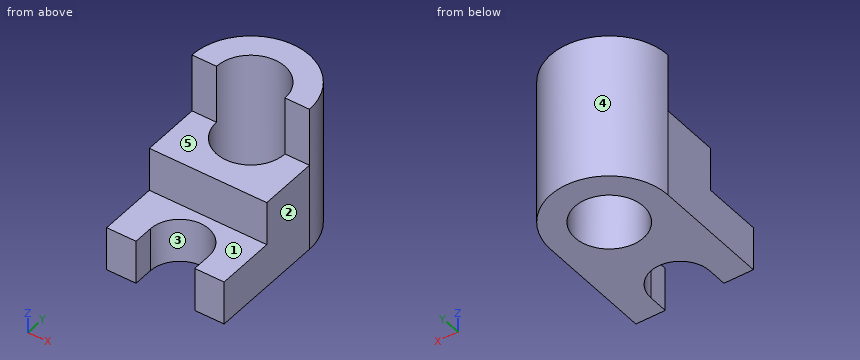
```python
from build123d import *

# Parameters (mm, degrees)
SKETCH1_R           = 3.5
BOSS_EXTRUDE1_DEPTH = 15
CUT_EXTRUDE1_DEPTH  = 15


with BuildPart() as part:
    # Sketch1 → Boss-Extrude1 (new body)
    with BuildSketch(Plane.XY):
        with BuildLine():
            Line((-6, 6), (-6, -6))
            Line((-6, -6), (-3, -6))
            Line((-3, -6), (-3, -3.996197441))
            ThreePointArc((-3, -3.996197441), (0, -0.996197441), (3, -3.996197441))
            Line((3, -3.996197441), (3, -6))
            Line((3, -6), (6, -6))
            Line((6, -6), (6, 6))
            ThreePointArc((6, 6), (0, 12), (-6, 6))
        make_face()
        with Locations((0, 6)):
            Circle(SKETCH1_R, mode=Mode.SUBTRACT)
    extrude(amount=BOSS_EXTRUDE1_DEPTH)

    # Sketch2 → Cut-Extrude1 (cut)
    with BuildSketch(Plane.ZY.offset(6)):
        Polygon((4.5, -6), (4.5, 0), (9, 0), (9, 6), (15, 6), (15, -6), align=None)
    extrude(amount=-CUT_EXTRUDE1_DEPTH, mode=Mode.SUBTRACT)


solid = part.part
```
Here's how the part is built. I have some questions about the finished solid (model axes, mm). Face numbers are marked on the shaded views. A direction names the side the tool comes from. Round coordinates to 2 decimals unless told otherwise and drop trailing zeros. Order: outer loops, then holes, each group sorted by start corner. A loop starts at its lowest first (then second) coordinate and runs counter-clockwise, first axis right, second up. Notation, with made-up numbers: M -20,34.5 L 10,34.5 A13 ccw 10,54.5 Z; hole C 2,58.25 d8. An arc over 180 degrees is marked long. Use CSV: the item, a comma, the result in double quotes.
1) I want a section at A-A (x = 0). List the corners of the cut face in (y, z) for me, then the cut area to 3 significant figures.
Taken from the geometry:
outline,"M -1,0 L 2.5,0 L 2.5,9 L 0,9 L 0,4.5 L -1,4.5 Z; M 9.5,0 L 12,0 L 12,15 L 9.5,15 Z"
area,"64.5 mm^2"
2) I need wall thicknesses on line 1 along Y through (x, z) = (0, 3.5); line 2 along Y through (x, z) = (0, 7); line 3 along X through (y, z) = (6, 3.75). Which ranges of each line are inside material? Lowest first, please. Write a range as [from, to].
Taken from the geometry:
line 1,"[-1, 2.5], [9.5, 12]"
line 2,"[0, 2.5], [9.5, 12]"
line 3,"[-6, -3.5], [3.5, 6]"
3) I want a section at D-D (z = 3). List the corners of the cut face in (x, y) for me.
Taken from the geometry:
outline,"M -6,-6 L -3,-6 L -3,-4 A3 cw 3,-4 L 3,-6 L 6,-6 L 6,6 A6 ccw -6,6 Z; hole C 0,6 d7"
4) I want a section at C-C (y = 9). List the corners of the cut face in (x, z) for me.
Taken from the geometry:
outline,"M -5.2,0 L -1.8,0 L -1.8,15 L -5.2,15 Z; M 1.8,0 L 5.2,0 L 5.2,15 L 1.8,15 Z"
5) I want a section at B-B (z = 7). List the corners of the cut face in (x, y) for me, then the cut area to 3 significant figures.
Taken from the geometry:
outline,"M -6,0 L 6,0 L 6,6 A6 ccw -6,6 Z; hole C 0,6 d7"
area,"90.1 mm^2"
6) I'm going to push flat-ended pins straight in: P1, Ø1.2, axis at x = 5, z = 12.5, coming from the -Y side; P2, Ø2, axis at x = 3, z = 8.5, coming from the +Y side; P3, Ø3, axis at y = 8.5, z = 12, coming from the +X side. Where does each tip first touch, or does it pass through?
Taken from the geometry:
P1,"y = 6"
P2,"y = 11.66"
P3,"x = 5.92"
7) If we mould it in two halves opening along X, with no side actions, what happens to the marked faces 1, 2 and 3? For each: pulls with the +X half, pulls with the -X half, needs draft (parallel to the pull), parting line crosses it, or undercut.
Taken from the geometry:
face 1,"needs draft"
face 2,"pulls with the +X half"
face 3,"undercut"
8) On a 3-axis mill with a long thin cutter (end or side, diameter ignored), from which of +Z, -Z, +X, -X, +Y, -Y can I reach the whole of each face in a straight line? I mean the marked faces 4 and 5. Say none if no direction works.
Taken from the geometry:
face 4,"+Z, -Z, +Y"
face 5,"+Z, +X, -X, -Y"
